Design review of the part built by this model. Coordinates are the model's own, in mm. Face numbers are marked on the shaded views. A direction names the side the tool comes from. Give positions to 0.01 mm unless a question says otherwise; leave off trailing zeros. Write each loop counter-clockwise with the first axis right and the second up, starting at its lowest first coordinate (ties: lowest second). Pieces come first, ordered by that corner, then holes. Notation, with made-up numbers: (78, -5.75) -> (105, -5.75) arc R26 cw to (105, 22.25) -> close; hole circle Ø4 at (-11, 39.5). An arc over 180 degrees is marked (long way). Return JSON: item names as keys, results as strings. Group by question number.
from build123d import *

# Parameters (mm, degrees)
ESBO_O1_R                     = 7.5
RESSALTO_EXTRUS_O1_DEPTH      = 8
ESBO_O2_R                     = 8.5
RESSALTO_EXTRUS_O2_DEPTH      = 3
ESBO_O3_W                     = 8
ESBO_O3_H                     = 3
RESSALTO_EXTRUS_O3_DEPTH      = 10
CORTE_EXTRUS_O1_DEPTH         = 23.27666941
CORTE_EXTRUS_O1_DEPTH_BACK    = 23.27666941
ESBO_O5_R                     = 3
CORTE_EXTRUS_O2_DEPTH         = 3
ESBO_O6_R                     = 5.5
RESSALTO_EXTRUS_O4_DEPTH      = 10
FILETE1_R                     = 1
ESBO_O8_R                     = 1.75
RESSALTO_EXTRUS_O5_DEPTH      = 10
ESBO_O10_R                    = 4.5
RESSALTO_EXTRUS_O6_DEPTH      = 3.5
ESBO_O11_W                    = 5
ESBO_O11_H                    = 3
RESSALTO_EXTRUS_O7_DEPTH      = 5
RESSALTO_EXTRUS_O8_DEPTH      = 1.5
RESSALTO_EXTRUS_O8_DEPTH_BACK = 1.5
ESBO_O13_R                    = 4
ESBO_O14_R                    = 2.5
CORTE_EXTRUS_O3_DEPTH         = 10
FILETE2_R                     = 10
FILETE3_R                     = 3
CUT_EXTRUDE2_START            = -24
CUT_EXTRUDE2_OUTLINE_R        = 8.5
CUT_EXTRUDE2_DEPTH            = 43
SKETCH2_R                     = 2.5
SKETCH2_R_2                   = 1.5
BOSS_EXTRUDE1_DEPTH           = 3


with BuildPart() as part:
    # Esboço1 → Ressalto-extrusão1 (new body)
    with BuildSketch(Plane(origin=(0, 0, 0), x_dir=(1, 0, 0), z_dir=(0, 1, 0))):
        with Locations(Location((0, 0, 0), (0, 0, 270))):
            Circle(ESBO_O1_R)
    extrude(amount=RESSALTO_EXTRUS_O1_DEPTH)

    # Esboço2 → Ressalto-extrusão2 (add)
    with BuildSketch(Plane.XZ):
        with Locations(Location((0, 0, 0), (0, 0, 270))):
            Circle(ESBO_O2_R)
    extrude(amount=RESSALTO_EXTRUS_O2_DEPTH)

    # Esboço3 → Ressalto-extrusão3 (add)
    with BuildSketch(Plane(origin=(0, 8, 0), x_dir=(1, 0, 0), z_dir=(0, 1, 0))):
        Rectangle(ESBO_O3_W, ESBO_O3_H)
    extrude(amount=RESSALTO_EXTRUS_O3_DEPTH)

    # Esboço4 → Corte-extrusão1 (cut, two sides: drawn at the far end of the back side and taken through both)
    with BuildSketch(Plane.XY.offset(1.5).offset(-CORTE_EXTRUS_O1_DEPTH_BACK)):
        with BuildLine():
            Line((-4, 18), (-4, 13.999999871))
            ThreePointArc((-4, 13.999999871), (-2.828427176, 16.828427073), (-1.7e-08, 18))
            Line((-1.7e-08, 18), (-4, 18))
        make_face()
        with BuildLine():
            Line((4, 18), (-1.7e-08, 18))
            ThreePointArc((-1.7e-08, 18), (2.828427119, 16.828427131), (4, 14))
            Line((4, 14), (4, 18))
        make_face()
    extrude(amount=CORTE_EXTRUS_O1_DEPTH + CORTE_EXTRUS_O1_DEPTH_BACK, mode=Mode.SUBTRACT)

    # Esboço5 → Corte-extrusão2 (cut)
    with BuildSketch(Plane.XY.offset(1.5)):
        with Locations((0, 14)):
            Circle(ESBO_O5_R)
    extrude(amount=-CORTE_EXTRUS_O2_DEPTH, mode=Mode.SUBTRACT)

    # Esboço6 → Ressalto-extrusão4 (add)
    with BuildSketch(Plane.XZ.offset(3)):
        with Locations(Location((0, 0, 0), (0, 0, 270))):
            Circle(ESBO_O6_R)
    extrude(amount=RESSALTO_EXTRUS_O4_DEPTH)

    # Loft1: read off the stored shape, not the designer's step
    # Loft1: loft between two sections, ruled curve by curve
    loft1_from = [
        Edge.make_bspline([(1.054348973, -13, 5.397994835), (-9.741640698, -13, 7.506692781), (-11.850338644, -13, -3.28929689), (-1.054348973, -13, -5.397994835), (9.741640698, -13, -7.506692781), (11.850338644, -13, 3.28929689), (1.054348973, -13, 5.397994835)], [0, 0, 0, 0, 0.5, 0.5, 0.5, 1, 1, 1, 1], 3, [1, 0.333333333, 0.333333333, 1, 0.333333333, 0.333333333, 1]),
    ]
    loft1_to = [
        Edge.make_bspline([(-0.660465845, -24, 3.945096307), (-8.550658458, -24, 2.624164617), (-7.229726768, -24, -5.266027996), (0.660465845, -24, -3.945096307), (8.550658458, -24, -2.624164617), (7.229726768, -24, 5.266027996), (-0.660465845, -24, 3.945096307)], [0, 0, 0, 0, 0.5, 0.5, 0.5, 1, 1, 1, 1], 3, [1, 0.333333333, 0.333333333, 1, 0.333333333, 0.333333333, 1]),
    ]
    loft1 = Solid(Shell([*[Face.make_surface_from_curves(loft1_from[k], loft1_to[k]) for k in range(1)], Face(Wire(loft1_from)), Face(Wire(loft1_to))]))
    add(loft1)

    # Filete1
    filete1_edges = [part.edges().sort_by_distance(p)[0] for p in [
        (-5.474439314, -13, 0.529635915),
    ]]
    fillet(filete1_edges, radius=FILETE1_R)

    # Esboço8 → Ressalto-extrusão5 (add)
    with BuildSketch(Plane.XZ.offset(24)):
        with Locations(Location((0, 0, 0), (0, 0, 270))):
            Circle(ESBO_O8_R)
    extrude(amount=RESSALTO_EXTRUS_O5_DEPTH)

    # Esboço9 → Revolução1 (revolve)
    with BuildSketch(Plane(origin=(0, 0, 0), x_dir=(0, 0, -1), z_dir=(1, 0, 0)), mode=Mode.PRIVATE) as revolu_o1_sk:
        Polygon((0, -34), (6, -34), (8.480200039, -31.023759953), (8.5, -32), (6, -35), (0, -35), align=None)
    revolve(revolu_o1_sk.sketch.rotate(Axis((0, 0, 0), (0, -1, 0)), 180), axis=Axis((0, 0, 0), (0, -1, 0)))

    # Esboço10 → Ressalto-extrusão6 (add)
    with BuildSketch(Plane.XZ.offset(35)):
        with Locations(Location((0, 0, 0), (0, 0, 90))):
            Circle(ESBO_O10_R)
    extrude(amount=RESSALTO_EXTRUS_O6_DEPTH)

    # Esboço11 → Ressalto-extrusão7 (add)
    with BuildSketch(Plane.XZ.offset(38.5)):
        Rectangle(ESBO_O11_W, ESBO_O11_H)
    extrude(amount=RESSALTO_EXTRUS_O7_DEPTH)

    # Esboço13 → Ressalto-extrusão8 (add, two sides: drawn at the far end of the back side and taken through both)
    with BuildSketch(Plane.XY.offset(-RESSALTO_EXTRUS_O8_DEPTH_BACK)):
        with Locations((0.000453955, -45.999999998)):
            Circle(ESBO_O13_R)
    extrude(amount=RESSALTO_EXTRUS_O8_DEPTH + RESSALTO_EXTRUS_O8_DEPTH_BACK)

    # Esboço14 → Corte-extrusão3 (cut)
    with BuildSketch(Plane(origin=(0, 0, -1.5), x_dir=(-1, 0, 0), z_dir=(0, 0, -1))):
        with Locations((-0.000453955, -45.999999998)):
            Circle(ESBO_O14_R)
    extrude(amount=-CORTE_EXTRUS_O3_DEPTH, mode=Mode.SUBTRACT)

    # Filete2
    # the kernel refuses this fillet: 10 mm, written as the material it takes off along each edge
    with BuildSketch(Plane(origin=(0, -35, 0), x_dir=(0, 0, 1), z_dir=(1, 0, 0))) as filete2_piece_1:
        with BuildLine():
            CenterArc((0.686510113, -9.244311488), FILETE2_R, 39.805571092, 27.777161729)
            Line((4.5, 0), (6, 0))
            Line((6, 0), (8.368722909, -2.842467491))
        make_face()
    revolve(axis=Axis((0, -35, 0), (0, -1, 0)), mode=Mode.SUBTRACT)

    # Filete3
    filete3_edges = [part.edges().sort_by_distance(p)[0] for p in [
        (0, -34, -6),
    ]]
    fillet(filete3_edges, radius=FILETE3_R)

    # Cut-Extrude2: read off the stored shape, not the designer's step
    # Cut-Extrude2 outline → Cut-Extrude2 (cut)
    with BuildSketch(Plane(origin=(0, 0, 0), x_dir=(1, 0, 0), z_dir=(0, 1, 0)).offset(CUT_EXTRUDE2_START)):
        Circle(CUT_EXTRUDE2_OUTLINE_R)
    extrude(amount=CUT_EXTRUDE2_DEPTH, mode=Mode.SUBTRACT)

    # Sketch2 → Boss-Extrude1 (add)
    with BuildSketch(Plane(origin=(0, 0, -1.5), x_dir=(-1, 0, 0), z_dir=(0, 0, -1))):
        with Locations((-0.000453955, -45.999999998)):
            Circle(SKETCH2_R)
        with Locations(Location((-0.000453955, -45.999999998, 0), (0, 0, 90))):
            Circle(SKETCH2_R_2, mode=Mode.SUBTRACT)
    extrude(amount=-BOSS_EXTRUDE1_DEPTH)


solid = part.part
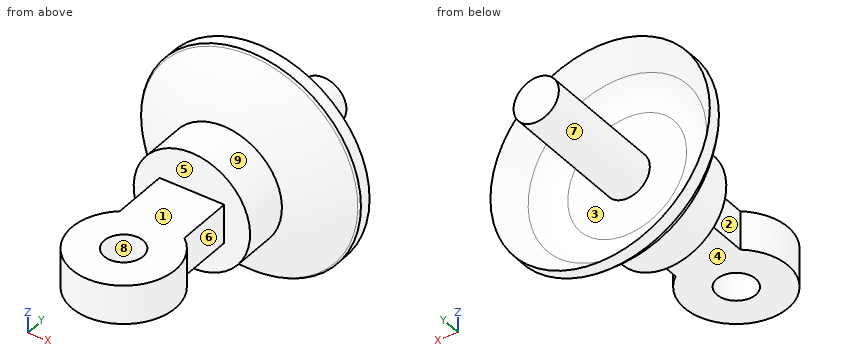
Q1. For L1, parallel to X at y = -46, z = 0.7; L2, parallel to X at y = -33.25, z = 0.25; L3, parallel to Y at x = -3.25, z = 1, list the stretches that pass through material, from the lowest coordinate up. Write a range as from..to.
Q2. Insertion check: pin 1 (1.8 mm diameter, centred on x = 0, y = -46, fed in from -Z); pin 2 (1.5 mm diameter, centred on x = 3, y = -45.5, fed in from +Z); pin 3 (2 mm diameter, centred on y = -43, z = 0.5, fed in from -X); pin 4 (6.5 mm diameter, centred on x = 1.5, y = -42, fed in from -Z). Each pin has a flat end and moves straight along its axis. Give the tip position at first contact, or say it passes through.
Q3. Mouldability with a two-part tool opening along X and no side actions: class the marked faces 6, 7, 8 and 9 as +X half, -X half, draft (parallel to the pull), parting line (faces both ways), or undercut.
Q4. Take a section at A-A, the plane y = -46. Give the boundary of the cut face in (x, z).
Q5. Take a section at B-B, the plane y = -26.5. Give the boundary of the cut face in (x, z), plus the area to 3 significant figures.
Q6. Take a section at C-C, the plane y = -40. Give the boundary of the cut face in (x, z), plus the area to 3 significant figures.
Q7. Take a section at D-D, the plane y = -35.75. Give the boundary of the cut face in (x, z).
Q8. Tool access review of the marked faces 1, 2, 3, 4 and 5: name each direction out of +Z, -Z, +X, -X, +Y, -Y from which nothing blocks a thin tool from reaching the whole face with its end or side.
Final values:
{
 "1": {"L1": "x = -4..-1.5, 1.5..4", "L2": "x = -7.3..-6.57, -1.73..1.73, 6.57..7.3", "L3": "y = -48.33..-43.67, -38.5..-34"},
 "2": {"pin 1": "passes through", "pin 2": "stops at z = 1.5", "pin 3": "stops at x = -3.46", "pin 4": "stops at z = -1.5"},
 "3": {"face 6": "+X half", "face 7": "undercut", "face 8": "undercut", "face 9": "parting line"},
 "4": {"outline": "(-4, -1.5) -> (-1.5, -1.5) -> (-1.5, 1.5) -> (-4, 1.5) -> close; (1.5, -1.5) -> (4, -1.5) -> (4, 1.5) -> (1.5, 1.5) -> close"},
 "5": {"outline": "circle Ø3.5 at (0, 0)", "area": "9.62 mm²"},
 "6": {"outline": "(-2.5, -1.5) -> (2.5, -1.5) -> (2.5, 1.5) -> (-2.5, 1.5) -> close", "area": "15.0 mm²"},
 "7": {"outline": "circle Ø9 at (0, 0)"},
 "8": {"face 1": "+Z, +X, -X, -Y", "face 2": "+Z, -Z, -X", "face 3": "+Y", "face 4": "-Z, +X, -X, -Y", "face 5": "none"}
}
